```python
from build123d import *

# Parameters (mm, degrees)
BOSS_EXTRUDE1_DEPTH               = 550
CHAMFER7_SIZE                     = 50.8
CHAMFER8_SIZE                     = 50.8
BOTTHOMHOLES_SKETCH2_R            = 12
BOTTHOMHOLES_SKETCH2_R_2          = 1.5875
BOTTOMHOLES_CUT_EXTRUDE1_DEPTH    = 553.788015993
RIGHTSIDEHOLES_SKETCH3_R          = 1.5875
RIGHTSIDEHOLES_CUT_EXTRUDE2_DEPTH = 553.924768843


with BuildPart() as part:
    # Sketch1 → Boss-Extrude1 (new body)
    with BuildSketch(Plane(origin=(0, 0, 0), x_dir=(0, 0, -1), z_dir=(1, 0, 0))):
        Polygon((0, 0), (-50.8, 0), (-50.8, 3.175), (-3.175, 3.175), (-3.175, 25.4), (0, 25.4), align=None)
    extrude(amount=BOSS_EXTRUDE1_DEPTH)

    # Chamfer7
    chamfer7_edges = [part.edges().sort_by_distance(p)[0] for p in [
        (0, 1.5875, 50.8),
    ]]
    chamfer(chamfer7_edges, length=CHAMFER7_SIZE - 0.0001)  # a hair under: the kernel refuses the full size

    # Chamfer8
    chamfer8_edges = [part.edges().sort_by_distance(p)[0] for p in [
        (550, 1.5875, 50.8),
    ]]
    chamfer(chamfer8_edges, length=CHAMFER8_SIZE - 0.0001)  # a hair under: the kernel refuses the full size

    # BotthomHoles-Sketch2 → BottomHoles-Cut-Extrude1 (cut, through all)
    with BuildSketch(Plane(origin=(0, 3.175, 0), x_dir=(1, 0, 0), z_dir=(0, 1, 0))):
        with Locations(Location((479.425, -24.175, 0), (0, 0, 270))):
            Circle(BOTTHOMHOLES_SKETCH2_R)
        with Locations(Location((463.925, -8.675, 0), (0, 0, 270))):
            Circle(BOTTHOMHOLES_SKETCH2_R_2)
        with Locations(Location((494.925, -8.675, 0), (0, 0, 270))):
            Circle(BOTTHOMHOLES_SKETCH2_R_2)
        with Locations(Location((463.925, -39.675, 0), (0, 0, 270))):
            Circle(BOTTHOMHOLES_SKETCH2_R_2)
        with Locations(Location((494.925, -39.675, 0), (0, 0, 270))):
            Circle(BOTTHOMHOLES_SKETCH2_R_2)
        with Locations(Location((39.6875, -11.1125, 0), (0, 0, 270))):
            Circle(BOTTHOMHOLES_SKETCH2_R_2)
        with Locations(Location((510.3125, -11.1125, 0), (0, 0, 270))):
            Circle(BOTTHOMHOLES_SKETCH2_R_2)
        with Locations(Location((178.925, -39.675, 0), (0, 0, 270))):
            Circle(BOTTHOMHOLES_SKETCH2_R_2)
        with Locations(Location((147.925, -39.675, 0), (0, 0, 270))):
            Circle(BOTTHOMHOLES_SKETCH2_R_2)
        with Locations(Location((178.925, -8.675, 0), (0, 0, 270))):
            Circle(BOTTHOMHOLES_SKETCH2_R_2)
        with Locations(Location((147.925, -8.675, 0), (0, 0, 270))):
            Circle(BOTTHOMHOLES_SKETCH2_R_2)
        with Locations(Location((163.425, -24.175, 0), (0, 0, 270))):
            Circle(BOTTHOMHOLES_SKETCH2_R)
    extrude(amount=-BOTTOMHOLES_CUT_EXTRUDE1_DEPTH, mode=Mode.SUBTRACT)

    # RightSideHoles-Sketch3 → RightSideHoles-Cut-Extrude2 (cut, through all)
    with BuildSketch(Plane(origin=(0, 0, 0), x_dir=(-1, 0, 0), z_dir=(0, 0, -1))):
        with Locations(Location((-529.3625, 17.4625, 0), (0, 0, 90))):
            Circle(RIGHTSIDEHOLES_SKETCH3_R)
        with Locations(Location((-538.8875, 11.1125, 0), (0, 0, 90))):
            Circle(RIGHTSIDEHOLES_SKETCH3_R)
        with Locations(Location((-529.3625, 11.1125, 0), (0, 0, 90))):
            Circle(RIGHTSIDEHOLES_SKETCH3_R)
        with Locations(Location((-11.1125, 11.1125, 0), (0, 0, 90))):
            Circle(RIGHTSIDEHOLES_SKETCH3_R)
        with Locations(Location((-20.6375, 11.1125, 0), (0, 0, 90))):
            Circle(RIGHTSIDEHOLES_SKETCH3_R)
        with Locations(Location((-20.6375, 17.4625, 0), (0, 0, 90))):
            Circle(RIGHTSIDEHOLES_SKETCH3_R)
        with Locations(Location((-412.5, 11.1125, 0), (0, 0, 90))):
            Circle(RIGHTSIDEHOLES_SKETCH3_R)
        with Locations(Location((-275, 11.1125, 0), (0, 0, 90))):
            Circle(RIGHTSIDEHOLES_SKETCH3_R)
        with Locations(Location((-137.5, 11.1125, 0), (0, 0, 90))):
            Circle(RIGHTSIDEHOLES_SKETCH3_R)
    extrude(amount=-RIGHTSIDEHOLES_CUT_EXTRUDE2_DEPTH, mode=Mode.SUBTRACT)


solid = part.part
```
Check sheet for the modelled part. Datum: model origin and axes. Units: mm. A direction names the side the tool comes from. Round coordinates to 2 decimals unless told otherwise and drop trailing zeros. Loops run counter-clockwise (first coordinate to the right, second up) from the corner with the lowest first, then second, coordinate; pieces in that order, holes last. Notation, with made-up numbers: (75, -26.5) -> (110, -26.5) arc R20 ccw to (110, -1.5) -> close; hole circle Ø7 at (83, 0). An arc over 180 degrees is marked (long way). Answer in a Markdown table with one row per item.
Q1. Release check for a two-part mould opening along X. For faces 1 (the face through (271, 13, 0)), 2 (the face through (173.54, 1.61, 30.63)), 3 (the face through (18, 2, 18)) record: released by +X, released by -X, zero draft, split by the parting line, or undercut.
Data:
| item | result |
|---|---|
| face 1 | zero draft |
| face 2 | undercut |
| face 3 | released by -X |
Q2. Sectioned sample at B-B on z = 31. Enter the section's corners in (x, y) (3 decimals), then the cut area to 3 significant figures.
Data:
| item | result |
|---|---|
| outline | (31, 0) -> (153.555, 0) -> (153.555, 3.175) -> (31, 3.175) -> close; (173.295, 0) -> (469.555, 0) -> (469.555, 3.175) -> (173.295, 3.175) -> close; (489.295, 0) -> (519, 0) -> (519, 3.175) -> (489.295, 3.175) -> close |
| area | 1,420 mm^2 |
Q3. Thickness scan on L1, parallel to X at y = 2.25, z = 26.5; L2, parallel to X at y = 2, z = 35; L3, parallel to Y at x = 71, z = 13 (3 decimals). Record the ranges inside material, lowest first.
Data:
| item | result |
|---|---|
| L1 | x = 26.5 to 151.65, 175.2 to 467.65, 491.2 to 523.5 |
| L2 | x = 35 to 158.25, 168.6 to 474.25, 484.6 to 515 |
| L3 | y = 0 to 3.175 |
Q4. Set-up check for faces 4 (the face through (491.323, 1.61, 22.613)), 5 (the face through (271, 14, 3.175)): record each of +Z, -Z, +X, -X, +Y, -Y from which the full face is reachable in a straight line by a thin tool's end or side.
Data:
| item | result |
|---|---|
| face 4 | +Y, -Y |
| face 5 | +Z, +X, -X, +Y |
Q5. Sectioned sample at A-A on x = 73. Enter the section's corners in (y, z) (3 decimals).
Data:
| item | result |
|---|---|
| outline | (0, 0) -> (25.4, 0) -> (25.4, 3.175) -> (3.175, 3.175) -> (3.175, 50.8) -> (0, 50.8) -> close |
Q6. Go/stop test with flat-tipped pins: P1, Ø5, axis at x = 137.5, y = 11.11, coming from the +Z side (3 decimals); P2, Ø1.9, axis at x = 147.925, z = 8.675, coming from the +Y side; P3, Ø3.5, axis at x = 463.925, z = 39.675, coming from the -Y side; P4, Ø4, axis at x = 324, z = 19.5, coming from the +Y side (3 decimals). Record where each tip stops, or that it passes through.
Data:
| item | result |
|---|---|
| P1 | stops at z = 3.175 |
| P2 | passes through |
| P3 | stops at y = 0 |
| P4 | stops at y = 3.175 |
